Design review of the part built by this model. Coordinates are the model's own, in mm. A direction names the side the tool comes from. Give positions to 0.01 mm unless a question says otherwise; leave off trailing zeros. Loops run counter-clockwise (first coordinate to the right, second up) from the corner with the lowest first, then second, coordinate; pieces in that order, holes last. Notation, with made-up numbers: M 52.5,34 L 103.5,34 A16 cw 103.5,44 Z; hole C 29.5,71.5 d3. An arc over 180 degrees is marked long. Answer as CSV lines item,"result".
Autodesk Inventor part; units mm, degrees
ref_plane "YZ Plane" through (0, 0, 0) normal (1, 0, 0) x (0, 1, 0)
ref_plane "XZ Plane" through (0, 0, 0) normal (0, 1, 0) x (-1, 0, 0)
ref_plane "XY Plane" through (0, 0, 0) normal (0, 0, 1) x (1, 0, 0)
sketch "Sketch1" plane through (0, 0, 0) normal (0, 0, 1) x (1, 0, 0)
  line L0 (-19.05, 38.1) -> (-14.2875, 38.1)
  line L1 (-14.2875, 38.1) -> (-14.2875, 4.7625)
  line L2 (-14.2875, 4.7625) -> (14.2875, 4.7625)
  line L3 (14.2875, 4.7625) -> (14.2875, 38.1)
  line L4 (14.2875, 38.1) -> (19.05, 38.1)
  line L5 (19.05, 38.1) -> (19.05, 0)
  line L6 (19.05, 0) -> (-19.05, 0)
  line L7 (-19.05, 0) -> (-19.05, 38.1)
  line L8 (0, 0) -> (0, 4.7625) construction
  dimension "d0" = 4.7625
  dimension "d2" = 38.1
  dimension "d3" = 38.1
extrude "Extrusion1" add sketch "Sketch1" along normal blind 73.025
sketch "Sketch2" plane through (-14.2875, 4.7625, 0) normal (0, 1, 0) x (1, 0, 0)
  line L0 (23.8125, -23.8125) -> (4.7625, -23.8125) construction
  line L1 (4.7625, -23.8125) -> (4.7625, -4.7625) construction
  line L2 (4.7625, -4.7625) -> (23.8125, -4.7625) construction
  line L3 (23.8125, -4.7625) -> (23.8125, -23.8125) construction
  line L4 (23.8125, -23.8125) -> (4.7625, -4.7625) construction
  line L5 (4.7625, -23.8125) -> (23.8125, -4.7625) construction
  circle A0 centre (4.7625, -4.7625) radius 2.54
  circle A1 centre (4.7625, -23.8125) radius 2.54
  circle A2 centre (23.8125, -4.7625) radius 2.54
  circle A3 centre (23.8125, -23.8125) radius 2.54
  line L6 (0, 0) -> (0, -73.025)
  line L7 (28.575, 0) -> (28.575, -73.025)
  line L8 (0, -73.025) -> (28.575, -73.025)
  line L9 (28.575, -73.025) -> (28.575, -28.575)
  line L10 (28.575, -28.575) -> (0, -28.575)
  line L11 (0, -28.575) -> (0, -73.025)
  line L12 (14.2875, -4.7625) -> (14.2875, 0) construction
  point P0 (14.2875, -14.2875)
  dimension "d6" = 5.08
  dimension "d7" = 19.05
  dimension "d8" = 19.05
  dimension "d10" = 14.2875
  dimension "d21" = 4.7625
  dimension "d22" = 4.7625
extrude "Extrusion2" cut sketch "Sketch2" against normal through all
sketch "Sketch3" plane through (19.05, 0, 0) normal (1, 0, 0) x (0, 0, -1)
  circle A0 centre (-52.3875, 19.05) radius 11.1125
  circle A1 centre (-52.3875, 19.05) radius 9.525 construction
  line L0 (-42.8625, 19.05) -> (-42.8625, -6.9181) construction
  line L1 (0, 0) -> (-73.025, 0) construction
  dimension "d15" = 19.05
  dimension "d13" = 22.225
  dimension "d14" = 19.05
  dimension "d16" = 42.8625
extrude "Extrusion3" cut sketch "Sketch3" against normal through all
fillet "Fillet1" radius 12.7 6 edges at (16.6687, 38.1, 73.025) (-16.6687, 38.1, 73.025) (16.6687, 38.1, 0) (-16.6687, 38.1, 0) (-16.6688, 0, 73.025) (16.6688, 0, 73.025)
properties part number "top pully bracket 2" material "Aluminum 6061"
1. We need section D-D, the plane z = 67. Write out the cut boundary in (x, y), plus the area to 3 significant figures.
Answer block:
outline,"M -19.05,1.9 L -14.29,1.9 L -14.29,36.2 L -19.05,36.2 Z; M 14.29,1.9 L 19.05,1.9 L 19.05,36.2 L 14.29,36.2 Z"
area,"327 mm²"
2. For P1, Ø2.5, axis at x = -2.5, y = 3, coming from the +Z side (3 decimals); P2, Ø4, axis at x = 3.5, z = 21.5, coming from the +Y side, all flat-tipped, find the tip position at first contact; note any pin that passes through.
Answer block:
P1,"z = 28.575"
P2,"y = 4.76"
3. We need section C-C, the plane z = 14. Write out the cut boundary in (x, y).
Answer block:
outline,"M -19.05,0 L 19.05,0 L 19.05,38.1 L 14.29,38.1 L 14.29,4.76 L -14.29,4.76 L -14.29,38.1 L -19.05,38.1 Z"
4. To check wall thickness, follow L1, parallel to X at y = 29, z = 45; L2, parallel to Y at x = 4, z = 3.5; L3, parallel to Z at x = 15, y = 13.5 (3 decimals). State the ranges of each line that lie inside material, in increasing order. Write a range as [from, to].
Answer block:
L1,"[-19.05, -14.29], [14.29, 19.05]"
L2,"[0, 4.76]"
L3,"[0, 42.76], [62.015, 73.025]"
5. For faces 1 (the flat face through (0, 2, 28.575)), 2 (the cylindrical face through (16.635, 3.622, 69.206)), list the 3-axis set-ups (+Z, -Z, +X, -X, +Y, -Y) from which the entire face can be reached by the end or side of a thin tool; tool diameter is ignored.
Answer block:
face 1,"+Z, +Y, -Y"
face 2,"+Z, +X, -X, -Y"
6. The part is to be moulded in two halves that separate along Z. For faces 3 (the cylindrical face through (-16.64, 34.28, 3.62)), 4 (the flat face through (0, 4.762, 14)), 5 (the flat face through (-17, 19, 73.025)), 6 (the cylindrical face through (7.51, 2.41, 25.36)), say which applies: pulls with the +Z half, pulls with the -Z half, needs draft (parallel to the pull), parting line crosses it, or undercut.
Answer block:
face 3,"pulls with the -Z half"
face 4,"needs draft"
face 5,"pulls with the +Z half"
face 6,"undercut"
7. We need section A-A, the plane y = 19.05. Count the separate pieces of the cut face and the enclosed holes in it, plus the area to 3 significant figures.
Answer block:
separate pieces,"4"
enclosed holes,"0"
area,"484 mm²"
